Part model, mm, in its own coordinate system. Face numbers are marked on the shaded views. A direction names the side the tool comes from. Round coordinates to 2 decimals unless told otherwise and drop trailing zeros. Write each loop counter-clockwise with the first axis right and the second up, starting at its lowest first coordinate (ties: lowest second). Pieces come first, ordered by that corner, then holes.
1) Which spindle directions (+Z, -Z, +X, -X, +Y, -Y) get a long thin tool onto all of the face, cutting with end or side? Do the marked faces 1 and 2. Say none if no direction does.
2) Flat gauge pins, fed straight in: pin 1 (8 mm diameter, centred on y = 18.5, z = 87, fed in from -X); pin 2 (4 mm diameter, centred on x = 25.5, z = 19, fed in from +Y); pin 3 (3 mm diameter, centred on x = -8, z = 89.5, fed in from +Y); pin 4 (11 mm diameter, centred on x = 0, y = 0, fed in from +Z). Where does each tip first touch, or does it go through?
3) Saw through at A-A on z = 85. Write the cut outline in (x, y).
4) Drill centre lines: L1, parallel to Y at x = 0, z = 165; L2, parallel to Y at x = 3, z = 122; L3, parallel to X at y = 7, z = -3. Where is each one in solid material? Low to high.
```python
from build123d import *

# Parameters (mm, degrees)
SKETCH1_R           = 32
BOSS_EXTRUDE1_DEPTH = 210
SKETCH2_R           = 34.5
BOSS_EXTRUDE2_DEPTH = 18
CHAMFER1_SIZE       = 10
CHAMFER1_SIZE2      = 6.745085168
SKETCH3_R           = 27.754914832
BOSS_EXTRUDE3_DEPTH = 5
SKETCH4_R           = 15
BOSS_EXTRUDE4_DEPTH = 10
SKETCH5_R           = 4.25
CUT_EXTRUDE1_DEPTH  = 854
CHAMFER2_SIZE       = 5
CHAMFER2_SIZE_2     = 13.025445323
SKETCH7_R           = 31.9
BOSS_EXTRUDE7_DEPTH = 10
CHAMFER3_SIZE       = 5
CHAMFER3_SIZE2      = 17.437072219
FILLET1_R           = 2
BOSS_EXTRUDE8_START = 10
SKETCH8_R           = 15
BOSS_EXTRUDE8_DEPTH = 10
CUT_EXTRUDE2_START  = -311
SKETCH9_R           = 4.25
CUT_EXTRUDE2_DEPTH  = 311


with BuildPart() as part:
    # Sketch1 → Boss-Extrude1 (new body)
    with BuildSketch(Plane.XY):
        Circle(SKETCH1_R)
    extrude(amount=BOSS_EXTRUDE1_DEPTH)

    # Sketch2 → Boss-Extrude2 (add)
    with BuildSketch(Plane.XY.offset(210)):
        Circle(SKETCH2_R)
    extrude(amount=BOSS_EXTRUDE2_DEPTH)

    # Chamfer1
    chamfer1_edges = [part.edges().sort_by_distance(p)[0] for p in [
        (-34.5, 0, 228),
    ]]
    chamfer1_side = [part.faces().sort_by_distance(p)[0] for p in [
        (-34.5, 0, 219),
    ]]
    chamfer(chamfer1_edges, length=CHAMFER1_SIZE, length2=CHAMFER1_SIZE2, reference=chamfer1_side[0])

    # Sketch3 → Boss-Extrude3 (add)
    with BuildSketch(Plane.XY.offset(228)):
        Circle(SKETCH3_R)
    extrude(amount=BOSS_EXTRUDE3_DEPTH)

    # Sketch4 → Boss-Extrude4 (add)
    with BuildSketch(Plane.XY.offset(233)):
        Circle(SKETCH4_R)
    extrude(amount=BOSS_EXTRUDE4_DEPTH)

    # Sketch5 → Cut-Extrude1 (cut)
    with BuildSketch(Plane.XY.offset(243)):
        Circle(SKETCH5_R)
    extrude(amount=-CUT_EXTRUDE1_DEPTH, mode=Mode.SUBTRACT)

    # Chamfer2
    # the kernel refuses this chamfer: 13.025445323, 5 mm, written as the material it takes off along each edge
    with BuildSketch(Plane(origin=(0, 0, 233), x_dir=(1, 0, 0), z_dir=(0, -1, 0))) as chamfer2_piece_1_section:
        Polygon((27.754914832, -CHAMFER2_SIZE), (27.754914832 - CHAMFER2_SIZE_2, 0), (27.754914832, 0), align=None)
    chamfer2_piece_1 = revolve(axis=Axis((0, 0, 233), (0, 0, 1)), mode=Mode.PRIVATE)
    chamfer2_piece_1 = chamfer2_piece_1 - Plane(origin=(0, 0, 228.02141562), x_dir=(1, 0, 0), z_dir=(0, 0, -1)) * Cylinder(15, 112, mode=Mode.PRIVATE)
    add(chamfer2_piece_1, mode=Mode.SUBTRACT)

    # Sketch7 → Boss-Extrude7 (add)
    with BuildSketch(Plane(origin=(0, 0, 0), x_dir=(-1, 0, 0), z_dir=(0, 0, -1))):
        with Locations(Location((0, 0, 0), (0, 0, 180))):
            Circle(SKETCH7_R)
    extrude(amount=BOSS_EXTRUDE7_DEPTH)

    # Chamfer3
    chamfer3_edges = [part.edges().sort_by_distance(p)[0] for p in [
        (-31.9, 0, -10),
    ]]
    chamfer3_side = [part.faces().sort_by_distance(p)[0] for p in [
        (-31.9, 0, -5),
    ]]
    chamfer(chamfer3_edges, length=CHAMFER3_SIZE, length2=CHAMFER3_SIZE2, reference=chamfer3_side[0])

    # Fillet1
    fillet1_edges = [part.edges().sort_by_distance(p)[0] for p in [
        (-31.9, 0, -5),
    ]]
    fillet(fillet1_edges, radius=FILLET1_R)

    # Sketch8 → Boss-Extrude8 (add)
    with BuildSketch(Plane(origin=(0, 0, -10), x_dir=(-1, 0, 0), z_dir=(0, 0, -1)).offset(BOSS_EXTRUDE8_START)):
        Circle(SKETCH8_R)
    extrude(amount=-BOSS_EXTRUDE8_DEPTH)

    # Sketch9 → Cut-Extrude2 (cut)
    with BuildSketch(Plane(origin=(0, 0, -20), x_dir=(-1, 0, 0), z_dir=(0, 0, -1)).offset(CUT_EXTRUDE2_START)):
        with Locations(Location((0, 0, 0), (0, 0, 180))):
            Circle(SKETCH9_R)
    extrude(amount=CUT_EXTRUDE2_DEPTH, mode=Mode.SUBTRACT)


solid = part.part
```
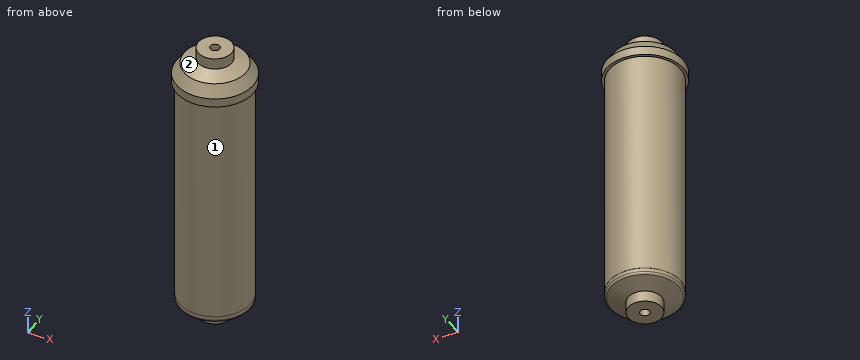
Completed:
1. face 1: -Z
1. face 2: +Z
2. pin 1: stops at x = -28.53
2. pin 2: stops at y = 21.72
2. pin 3: stops at y = 31.33
2. pin 4: stops at z = 243
3. outline: circle Ø64 at (0, 0); hole circle Ø8.5 at (0, 0)
4. L1: y = -32 to -4.25, 4.25 to 32
4. L2: y = -31.86 to -3.01, 3.01 to 31.86
4. L3: x = -31.12 to 31.12
